For this review, take the finished solid that the model builds, in its own axes (mm). Face numbers are marked on the shaded views. A direction names the side the tool comes from. Round coordinates to 2 decimals unless told otherwise and drop trailing zeros. Order: outer loops, then holes, each group sorted by start corner. A loop starts at its lowest first (then second) coordinate and runs counter-clockwise, first axis right, second up. Notation, with made-up numbers: M 7.25,4.25 L 17.25,4.25 A27 cw 17.25,34.25 Z; hole C -15.5,54 d2. An arc over 180 degrees is marked long. Use a Markdown table: item, result.
from build123d import *

# Parameters (mm, degrees)
EXTRUDE_1_DEPTH = 20
SKETCH_3_R      = 20
EXTRUDE_2_DEPTH = 20


with BuildPart() as part:
    # 草图2 → 凸台-拉伸1 (new body)
    with BuildSketch(Plane.XY):
        Polygon((50, 0), (-50, 0), (-50, -10), (-45, -10), (-20, -50), (-20, -10), (20, -10), (20, -50), (45, -10), (50, -10), align=None)
    extrude(amount=EXTRUDE_1_DEPTH)

    # 草图3 → 凸台-拉伸2 (add)
    with BuildSketch(Plane(origin=(0, 0, 0), x_dir=(1, 0, 0), z_dir=(0, 1, 0))):
        with Locations(Location((0, -10, 0), (0, 0, 30))):
            Circle(SKETCH_3_R)
    extrude(amount=EXTRUDE_2_DEPTH)


solid = part.part
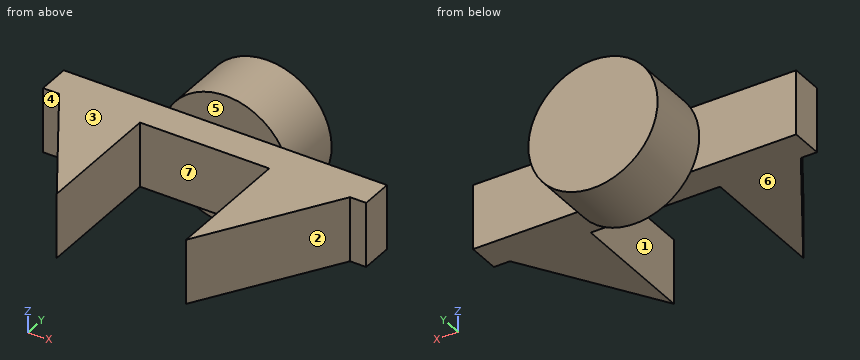
Q1. Add section A-A (y = -13). Write out the cut boundary in (x, z) (3 decimals), then the cut area to 3 significant figures.
Determined:
| item | result |
|---|---|
| outline | M -43.125,0 L -20,0 L -20,20 L -43.125,20 Z; M 20,0 L 43.125,0 L 43.125,20 L 20,20 Z |
| area | 925 mm^2 |
Q2. Add section C-C (x = 0). Write out the cut boundary in (y, z), then the cut area to 3 significant figures.
Determined:
| item | result |
|---|---|
| outline | M -10,0 L 0,0 L 0,-10 L 20,-10 L 20,30 L 0,30 L 0,20 L -10,20 Z |
| area | 1,000 mm^2 |
Q3. Machinability: for the marked faces 4, 5, 6 and 7, which of the approach directions +Z, -Z, +X, -X, +Y, -Y give a long, thin tool a straight path to every point of the face, cutting with its end or side? Answer none if there is none.
Determined:
| item | result |
|---|---|
| face 4 | +Z, -Z, -X, -Y |
| face 5 | +Z, +X, -X, -Y |
| face 6 | -Z, +X, -X, -Y |
| face 7 | +Z, -Z, -Y |
Q4. Clearance check with flat-ended pins moving along their axes: pin 1 (10 mm diameter, centred on x = 31, z = 11.5, fed in from +Y); pin 2 (16 mm diameter, centred on y = -38, z = 9, fed in from +X); pin 3 (10 mm diameter, centred on y = -25, z = 13.5, fed in from -X). State where each tip first meets the part, or that it passes through.
Determined:
| item | result |
|---|---|
| pin 1 | stops at y = 0 |
| pin 2 | stops at x = 32.5 |
| pin 3 | stops at x = -38.75 |
Q5. Add section D-D (y = 7). Write out the cut boundary in (x, z).
Determined:
| item | result |
|---|---|
| outline | C 0,10 d40 |
Q6. Add section B-B (z = 10). Write out the cut boundary in (x, y), then the cut area to 3 significant figures.
Determined:
| item | result |
|---|---|
| outline | M -50,-10 L -45,-10 L -20,-50 L -20,-10 L 20,-10 L 20,-50 L 45,-10 L 50,-10 L 50,0 L 20,0 L 20,20 L -20,20 L -20,0 L -50,0 Z |
| area | 2,800 mm^2 |
Q7. Wall thickness on line 1 along X through (y, z) = (-15, 0.5) (3 decimals); line 2 along X through (y, z) = (-45.5, 2); line 3 along Z through (x, y) = (-21.5, -12): over which ranges is each line inside the solid? List them lowest first. Write a range as [from, to].
Determined:
| item | result |
|---|---|
| line 1 | x = [-41.875, -20], [20, 41.875] |
| line 2 | x = [-22.81, -20], [20, 22.81] |
| line 3 | z = [0, 20] |
Q8. Draft analysis for pull direction X (two halves, no side actions). For the marked faces 1, 2 and 3, state which applies: pulls with the +X half, pulls with the -X half, needs draft (parallel to the pull), parting line crosses it, or undercut.
Determined:
| item | result |
|---|---|
| face 1 | undercut |
| face 2 | pulls with the +X half |
| face 3 | needs draft |
